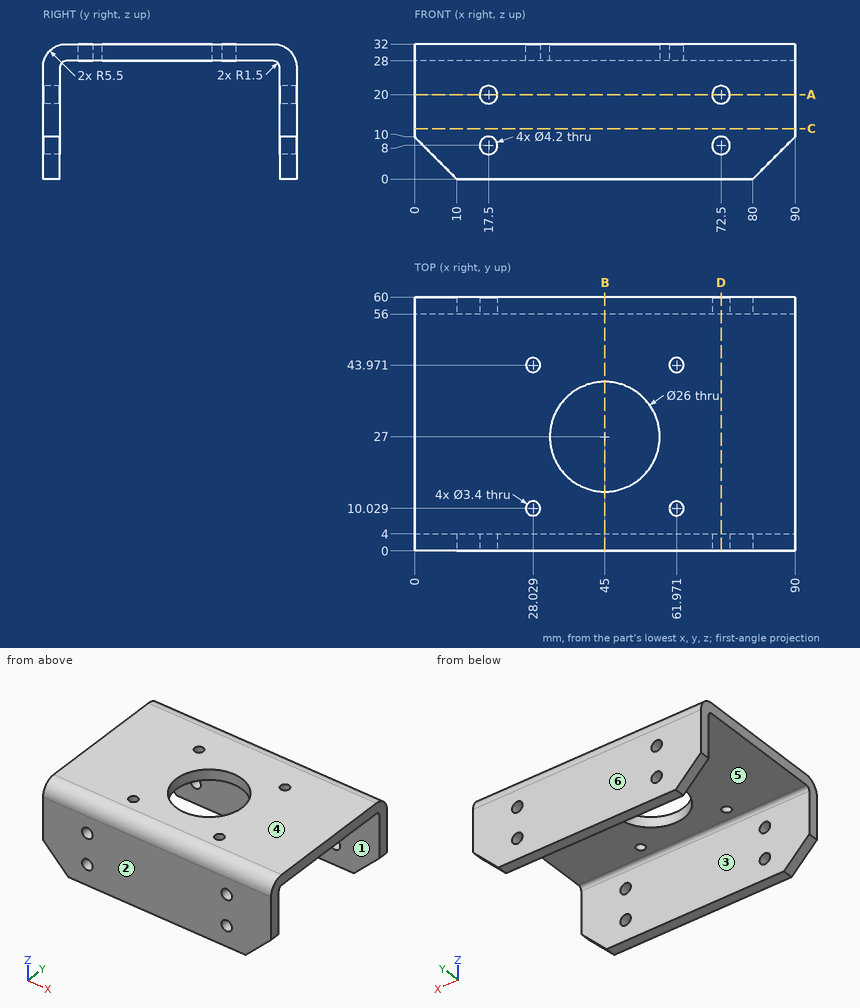
The figure shows three views and two pictorial views of one solid part (mm, origin at its lowest corner). Answer the questions. A direction names the side the tool comes from. Give positions to 0.01 mm unless a question says otherwise; leave off trailing zeros. Write each loop counter-clockwise with the first axis right and the second up, starting at its lowest first coordinate (ties: lowest second). Pieces come first, ordered by that corner, then holes.
Q1. The part is cut by section C-C on z = 12. Give the vertices of the cut face in (x, y).
Answer:
outline: (0, 0) - (90, 0) - (90, 4) - (0, 4) - close; (0, 56) - (90, 56) - (90, 60) - (0, 60) - close
Q2. A tool of negligible diameter and unlimited length cuts with its end or side. For the marked faces 5 and 6, from which of +Z, -Z, +X, -X, +Y, -Y can it reach the whole face along a straight path? Write none if from no direction.
Answer:
face 5: -Z, +X, -X
face 6: +Z, -Z, +X, -X, +Y
Q3. The part is cut by section A-A on z = 20. Give the vertices of the cut face in (x, y).
Answer:
outline: (0, 0) - (15.4, 0) - (15.4, 4) - (0, 4) - close; (0, 56) - (15.4, 56) - (15.4, 60) - (0, 60) - close; (19.6, 0) - (70.4, 0) - (70.4, 4) - (19.6, 4) - close; (19.6, 56) - (70.4, 56) - (70.4, 60) - (19.6, 60) - close; (74.6, 0) - (90, 0) - (90, 4) - (74.6, 4) - close; (74.6, 56) - (90, 56) - (90, 60) - (74.6, 60) - close
Q4. The part is cut by section D-D on x = 72.5. Give the vertices of the cut face in (y, z), and give its area (3 significant figures).
Answer:
outline: (0, 0) - (4, 0) - (4, 5.9) - (0, 5.9) - close; (0, 10.1) - (4, 10.1) - (4, 17.9) - (0, 17.9) - close; (0, 22.1) - (4, 22.1) - (4, 26.5) arc R1.5 cw to (5.5, 28) - (54.5, 28) arc R1.5 cw to (56, 26.5) - (56, 22.1) - (60, 22.1) - (60, 26.5) arc R5.5 ccw to (54.5, 32) - (5.5, 32) arc R5.5 ccw to (0, 26.5) - close; (56, 0) - (60, 0) - (60, 5.9) - (56, 5.9) - close; (56, 10.1) - (60, 10.1) - (60, 17.9) - (56, 17.9) - close
area: 385 mm2
Q5. The part is cut by section B-B on x = 45. Give the vertices of the cut face in (y, z), and give its area (3 significant figures).
Answer:
outline: (0, 0) - (4, 0) - (4, 26.5) arc R1.5 cw to (5.5, 28) - (14, 28) - (14, 32) - (5.5, 32) arc R5.5 ccw to (0, 26.5) - close; (40, 28) - (54.5, 28) arc R1.5 cw to (56, 26.5) - (56, 0) - (60, 0) - (60, 26.5) arc R5.5 ccw to (54.5, 32) - (40, 32) - close
area: 348 mm2
Q6. Given pin 1 (2 mm diameter, centred on x = 61.97, y = 10.03, fed in from +Z); pin 2 (5 mm diameter, centred on x = 51, y = 17.5, fed in from -Z); pin 3 (3 mm diameter, centred on x = 53.5, z = 26, fed in from -Y), each flat-ended and moving along its own axis, determine where each tip first touches the part or whether it passes through.
Answer:
pin 1: passes through
pin 2: stops at z = 28
pin 3: stops at y = 0
Q7. Straight lines are drawn through the part: L1, parallel to X at y = 2, z = 20; L2, parallel to Y at x = 4, z = 22; L3, parallel to Z at x = 17, y = 58. For each, find the intervals that lie inside material, in ascending order.
Answer:
L1: x = 0 to 15.4, 19.6 to 70.4, 74.6 to 90
L2: y = 0 to 4, 56 to 60
L3: z = 0 to 5.96, 10.04 to 17.96, 22.04 to 30.74
Q8. For a pull along Y with two mould halves and no side action, classify the marked faces 1, 2, 3 and 4 as released by +Y, released by -Y, zero draft, split by the parting line, or undercut.
Answer:
face 1: undercut
face 2: released by -Y
face 3: undercut
face 4: zero draft
